```python
from build123d import *

# Parameters (mm, degrees)
SKETCH1_R          = 20
BASE_EXTRUDE_DEPTH = 3


with BuildPart() as part:
    # Sketch1 → Base-Extrude (new body)
    with BuildSketch(Plane.XY):
        with Locations(Location((0, 0, 0), (0, 0, 180))):
            Circle(SKETCH1_R)
        with BuildLine():
            Line((1.944214305, 5), (12.373449734, 5))
            ThreePointArc((12.373449734, 5), (-13.345495806, 0), (12.373449734, -5))
            Line((12.373449734, -5), (1.944214305, -5))
            ThreePointArc((1.944214305, -5), (-1.64638645, -4.369036915), (-3.895643079, -1.5))
            Line((-3.895643079, -1.5), (4.736201703, -1.5))
            Line((4.736201703, -1.5), (4.736201703, 1.5))
            Line((4.736201703, 1.5), (-3.895643079, 1.5))
            ThreePointArc((-3.895643079, 1.5), (-1.64638645, 4.369036915), (1.944214305, 5))
        make_face(mode=Mode.SUBTRACT)
    extrude(amount=BASE_EXTRUDE_DEPTH)


solid = part.part
```
Could you check a few things on this model? Use its own coordinates, in mm. A direction names the side the tool comes from. Coordinates: 2 decimals unless noted, no trailing zeros. Loops run counter-clockwise (first coordinate to the right, second up) from the corner with the lowest first, then second, coordinate; pieces in that order, holes last. Notation, with made-up numbers: M 87,87 L 114,87 A15 cw 114,104 Z; hole C 63,70 d3. An arc over 180 degrees is marked long. Put each result on its own line as item: value. Start each with the question number.
(1) Thinking about a two-plate mould opening in Y: for faces 1 (the face through (19.98, -0.88, 1.48)), 2 (the face through (-1.601, -4.396, 1.479)), 3 (the face through (0, 4, 3)), which applies, pulls with the +Y half, pulls with the -Y half, needs draft (parallel to the pull), parting line crosses it, or undercut?
(2) For faces 4 (the face through (0, 4, 0)), 5 (the face through (4.736, 0, 1)), which set-ups out of +Z, -Z, +X, -X, +Y, -Y let a thin tool reach every point of the face, with its end or its side?
(3) Suppose I cut it at C-C on x = 0. Please give me the cut outline in (y, z).
(4) Suppose I cut it at B-B on z = 2.55. Please give me the cut outline in (x, y).
(5) I need wall thicknesses on line 1 (Y direction, x = 0, z = 2.3); line 2 (Y direction, x = 5, z = 1.3); line 3 (Y direction, x = 12, z = 2.35). Which ranges of each line are inside material? Lowest first, please. Write a range as from..to.
(6) Suppose I cut it at D-D on x = -11.5. Please give me the cut outline in (y, z).
(7) Suppose I cut it at A-A on y = 0. Please give me the cut outline in (x, z).
(8) Will these pins go through, and if not, where does the flat tip stop? P1, Ø1, axis at y = 1.5, z = 1.5, coming from the +X side (3 decimals); P2, Ø1.5, axis at y = -5.5, z = 0.5, coming from the +X side; P3, Ø8, axis at x = -5, y = 4, coming from the -Z side; P4, Ø1.5, axis at x = 0, z = 1, coming from the +Y side.
Solutions:
1. face 1: parting line crosses it
1. face 2: undercut
1. face 3: needs draft
2. face 4: -Z, +X, -X, +Y, -Y
2. face 5: +Z, -Z
3. outline: M -20,0 L -13.35,0 L -13.35,3 L -20,3 Z; M -5,0 L -1.5,0 L -1.5,3 L -5,3 Z; M 1.5,0 L 5,0 L 5,3 L 1.5,3 Z; M 13.35,0 L 20,0 L 20,3 L 13.35,3 Z
4. outline: C 0,0 d40; hole M -3.9,-1.5 L 4.74,-1.5 L 4.74,1.5 L -3.9,1.5 A5.09 cw 1.94,5 L 12.37,5 A13.35 ccw long 12.37,-5 L 1.94,-5 A5.09 cw Z
5. line 1: y = -20..-13.35, -5..-1.5, 1.5..5, 13.35..20
5. line 2: y = -19.36..-12.37, -5..5, 12.37..19.36
5. line 3: y = -16..-5.84, -5..5, 5.84..16
6. outline: M -16.36,0 L -6.77,0 L -6.77,3 L -16.36,3 Z; M 6.77,0 L 16.36,0 L 16.36,3 L 6.77,3 Z
7. outline: M -20,0 L -13.35,0 L -13.35,3 L -20,3 Z; M 4.74,0 L 20,0 L 20,3 L 4.74,3 Z
8. P1: stops at x = 19.975
8. P2: stops at x = 19.43
8. P3: stops at z = 0
8. P4: stops at y = 20
